Can you work these out from the model? Positions are in its coordinate system, mm. A direction names the side the tool comes from. Coordinates: 2 decimals unless noted, no trailing zeros. Order: outer loops, then holes, each group sorted by start corner. A loop starts at its lowest first (then second) coordinate and runs counter-clockwise, first axis right, second up. Notation, with made-up numbers: M 73,3 L 96,3 A16 ccw 96,32 Z; hole C 57,0 d4. An arc over 180 degrees is marked long. Answer as CSV lines item,"result". Start each with the question number.
1. I need wall thicknesses on line 1 along X through (y, z) = (0.3, -1.05); line 2 along Y through (x, z) = (-32, -1.65). Which ranges of each line are inside material? Lowest first, please. Write a range as from..to.
2. On a 3-axis mill with a long thin cutter (end or side, diameter ignored), from which of +Z, -Z, +X, -X, +Y, -Y can I reach the whole of each face in a straight line? I mean faces 1 (the face through (-1, 1.75, -2)), 2 (the face through (-5, 0, -2)). Say none if no direction works.
3. If we section it at B-B (z = -4.25): List the corners of the cut face in (x, y) for me.
4. If we section it at A-A (y = 0.6): List the corners of the cut face in (x, z) for me.
5. Will this pin go through, and if not, where does the flat tip stop? pin 1 (0.8 mm diameter, centred on x = -2, z = -2, fed in from +Y).
Autodesk Inventor part; units mm, degrees
ref_plane "YZ Plane" through (0, 0, 0) normal (1, 0, 0) x (0, 1, 0)
ref_plane "XZ Plane" through (0, 0, 0) normal (0, 1, 0) x (-1, 0, 0)
ref_plane "XY Plane" through (0, 0, 0) normal (0, 0, 1) x (1, 0, 0)
sketch "Sketch1" plane through (0, 0, 0) normal (0, 1, 0) x (-1, 0, 0)
  line L0 (0, 0) -> (36, 0)
  line L1 (36, 0) -> (36, -5)
  line L2 (36, -5) -> (0, -5)
  line L3 (0, -5) -> (0, 0)
  line L4 (0, 0) -> (1.5, 0)
  line L5 (1.5, 0) -> (1.5, -5)
  line L6 (1.5, -5) -> (0, -5)
  line L7 (0, -5) -> (0, 0)
  line L8 (1.5, -5) -> (3, -5)
  line L9 (3, -5) -> (3, 0)
  line L10 (3, 0) -> (1.5, 0)
  line L11 (1.5, 0) -> (1.5, -5)
  line L12 (3, 0) -> (4.5, 0)
  line L13 (4.5, 0) -> (4.5, -5)
  line L14 (4.5, -5) -> (3, -5)
  line L15 (3, -5) -> (3, 0)
  line L16 (4.5, -5) -> (6, -5)
  line L17 (6, -5) -> (6, 0)
  line L18 (6, 0) -> (4.5, 0)
  line L19 (4.5, 0) -> (4.5, -5)
  line L20 (36, -5) -> (32.5, -5)
  line L21 (32.5, -5) -> (32.5, 0)
  line L22 (32.5, 0) -> (36, 0)
  line L23 (36, 0) -> (36, -5)
  line L24 (32.5, 0) -> (29, 0)
  line L25 (29, 0) -> (29, -5)
  line L26 (29, -5) -> (32.5, -5)
  line L27 (32.5, -5) -> (32.5, 0)
  dimension "d0" = 36
  dimension "d1" = 5
  dimension "d2" = 1.5
  dimension "d3" = 1.5
  dimension "d4" = 1.5
  dimension "d5" = 1.5
  dimension "d6" = 3.5
  dimension "d7" = 3.5
extrude "Extrusion1" add sketch "Sketch1" along normal blind 1.75 contours L0 L5 L2 L3 | L0 L13 L2 L9 | L0 L25 L2 L17 | L0 L1 L2 L21
extrude "Extrusion2" add sketch "Sketch1" against normal blind 1.75
properties part number "Wall Test"
Solved:
1,line 1,"-36..-32.5, -29..-6, -4.5..-3, -1.5..0"
1,line 2,"-1.75..0"
2,face 1,"+Z, -Z, +X, -X, +Y"
2,face 2,"+Z, -Z, +Y"
3,outline,"M -36,-1.75 L 0,-1.75 L 0,1.75 L -1.5,1.75 L -1.5,0 L -3,0 L -3,1.75 L -4.5,1.75 L -4.5,0 L -6,0 L -6,1.75 L -29,1.75 L -29,0 L -32.5,0 L -32.5,1.75 L -36,1.75 Z"
4,outline,"M -36,-5 L -32.5,-5 L -32.5,0 L -36,0 Z; M -29,-5 L -6,-5 L -6,0 L -29,0 Z; M -4.5,-5 L -3,-5 L -3,0 L -4.5,0 Z; M -1.5,-5 L 0,-5 L 0,0 L -1.5,0 Z"
5,pin 1,"y = 0"
